from build123d import *

# Parameters (mm, degrees)
F1_DEPTH = 2
F2_DEPTH = 19
F3_R     = 2.75
F3_R_2   = 1.25
F4_DEPTH = 5
F5_W     = 9
F5_H     = 2
F5_W_2   = 17
F5_W_3   = 8
F5_W_4   = 2
F5_H_2   = 15.9
F5_H_3   = 15.1
F6_DEPTH = 12
F7_W     = 15.6
F7_H     = 4
F8_DEPTH = 2


with BuildPart() as f1:
    # F0 (on Top) → F1 (new body)
    with BuildSketch(Plane.XY):
        with BuildLine():
            ThreePointArc((0, 2.5), (0.732233047, 0.732233047), (2.5, 0))
            Line((2.5, 0), (88.5, 0))
            ThreePointArc((88.5, 0), (90.267766953, 0.732233047), (91, 2.5))
            Line((91, 2.5), (91, 59.5))
            ThreePointArc((91, 59.5), (90.267766953, 61.267766953), (88.5, 62))
            Line((88.5, 62), (2.5, 62))
            ThreePointArc((2.5, 62), (0.732233047, 61.267766953), (0, 59.5))
            Line((0, 59.5), (0, 2.5))
        make_face()
        with BuildLine():
            ThreePointArc((2, 59.5), (2.1464466094, 59.8535533906), (2.5, 60))
            Line((2.5, 60), (88.5, 60))
            ThreePointArc((88.5, 60), (88.8535533906, 59.8535533906), (89, 59.5))
            Line((89, 59.5), (89, 2.5))
            ThreePointArc((89, 2.5), (88.8535533906, 2.1464466094), (88.5, 2))
            Line((88.5, 2), (2.5, 2))
            ThreePointArc((2.5, 2), (2.1464466094, 2.1464466094), (2, 2.5))
            Line((2, 2.5), (2, 59.5))
        make_face(mode=Mode.SUBTRACT)
        with BuildLine():
            Line((88.5, 60), (2.5, 60))
            ThreePointArc((2.5, 60), (2.1464466094, 59.8535533906), (2, 59.5))
            Line((2, 59.5), (2, 2.5))
            ThreePointArc((2, 2.5), (2.1464466094, 2.1464466094), (2.5, 2))
            Line((2.5, 2), (88.5, 2))
            ThreePointArc((88.5, 2), (88.8535533906, 2.1464466094), (89, 2.5))
            Line((89, 2.5), (89, 59.5))
            ThreePointArc((89, 59.5), (88.8535533906, 59.8535533906), (88.5, 60))
        make_face()
    extrude(amount=F1_DEPTH)

    # F0 (on Top) → F2 (join)
    with BuildSketch(Plane.XY):
        with BuildLine():
            ThreePointArc((0, 2.5), (0.732233047, 0.732233047), (2.5, 0))
            Line((2.5, 0), (88.5, 0))
            ThreePointArc((88.5, 0), (90.267766953, 0.732233047), (91, 2.5))
            Line((91, 2.5), (91, 59.5))
            ThreePointArc((91, 59.5), (90.267766953, 61.267766953), (88.5, 62))
            Line((88.5, 62), (2.5, 62))
            ThreePointArc((2.5, 62), (0.732233047, 61.267766953), (0, 59.5))
            Line((0, 59.5), (0, 2.5))
        make_face()
        with BuildLine():
            ThreePointArc((2, 59.5), (2.1464466094, 59.8535533906), (2.5, 60))
            Line((2.5, 60), (88.5, 60))
            ThreePointArc((88.5, 60), (88.8535533906, 59.8535533906), (89, 59.5))
            Line((89, 59.5), (89, 2.5))
            ThreePointArc((89, 2.5), (88.8535533906, 2.1464466094), (88.5, 2))
            Line((88.5, 2), (2.5, 2))
            ThreePointArc((2.5, 2), (2.1464466094, 2.1464466094), (2, 2.5))
            Line((2, 2.5), (2, 59.5))
        make_face(mode=Mode.SUBTRACT)
    extrude(amount=F2_DEPTH)

    # F3 (on face) → F4 (join)
    with BuildSketch(Plane.XY.offset(2)):
        with Locations((6.5, 55.5)):
            Circle(F3_R)
        with Locations((6.5, 55.5)):
            Circle(F3_R_2, mode=Mode.SUBTRACT)
        with Locations((64.5, 55.5)):
            Circle(F3_R)
        with Locations((64.5, 55.5)):
            Circle(F3_R_2, mode=Mode.SUBTRACT)
        with Locations((6.5, 6.5)):
            Circle(F3_R)
        with Locations((6.5, 6.5)):
            Circle(F3_R_2, mode=Mode.SUBTRACT)
        with Locations((64.5, 6.5)):
            Circle(F3_R)
        with Locations((64.5, 6.5)):
            Circle(F3_R_2, mode=Mode.SUBTRACT)
    extrude(amount=F4_DEPTH)

    # F5 (on face) → F6 (cut)
    with BuildSketch(Plane.XY.offset(19)):
        with Locations((13.55, 1)):
            Rectangle(F5_W, F5_H)
        with Locations((35, 1)):
            Rectangle(F5_W_2, F5_H)
        with Locations((57.25, 1)):
            Rectangle(F5_W_3, F5_H)
        with Locations((90, 13.25)):
            Rectangle(F5_W_4, F5_H_2)
        with Locations((90, 30.95)):
            Rectangle(F5_W_4, F5_H_3)
        with Locations((90, 49.95)):
            Rectangle(F5_W_4, F5_H_3)
    extrude(amount=-F6_DEPTH, mode=Mode.SUBTRACT)

    # F7 (on face) → F8 (cut)
    with BuildSketch(Plane(origin=(0, 0, 0), x_dir=(0, -1, 0), z_dir=(-1, 0, 0))):
        with Locations((-31.7, 6)):
            Rectangle(F7_W, F7_H)
    extrude(amount=-F8_DEPTH, mode=Mode.SUBTRACT)


solid = f1.part
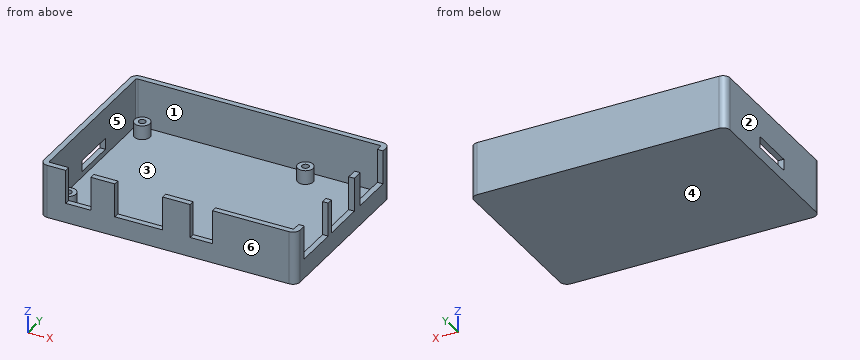
Read the model definition and answer for the solid it produces. Units are mm, in the model's axes. Face numbers are marked on the shaded views. A direction names the side the tool comes from. Give positions to 0.01 mm unless a question says otherwise; leave off trailing zeros. Write each loop counter-clockwise with the first axis right and the second up, starting at its lowest first coordinate (ties: lowest second). Pieces come first, ordered by that corner, then holes. Notation, with made-up numbers: (77.5, 77) -> (98.5, 77) arc R36 cw to (98.5, 111) -> close; hole circle Ø10 at (-7.75, 33). An arc over 180 degrees is marked (long way). Answer as a JSON object with one key per item and string values. Group by question number.
1) Find section A-A (y = 6.5). Write down the section's boundary in (x, z), and give its area (3 significant figures).
2) Each of these flat-tipped pins is pushed along its axis until it touches: P1, Ø2, axis at x = 35.5, y = 1, coming from the +Z side; P2, Ø1, axis at x = 90.5, z = 14.5, coming from the -Y side; P3, Ø0.6, axis at x = 89.5, z = 12, coming from the +Y side. Where does it stop, or does it pass through?
3) Find section D-D (y = 19.5). Write down the section's boundary in (x, z), and give its area (3 significant figures).
4) Consider L1, parallel to Y at x = 6.5, z = 4.8; L2, parallel to Y at x = 74, z = 2.5; L3, parallel to X at y = 58.5, z = 14.25. Determine where each line is inside the solid, lowest interval first. Write a range as from..to.
5) Find section B-B (x = 64.5). Write down the section's boundary in (y, z).
6) The mould has two halves that part along X. Classify the marked faces 1, 2, 3 and 4: +X half, -X half, draft (parallel to the pull), parting line (faces both ways), or undercut.
7) A tool of negligible diameter and unlimited length cuts with its end or side. For the marked faces 5 and 6, from which of +Z, -Z, +X, -X, +Y, -Y can it reach the whole face along a straight path? Write none if from no direction.
8) Find section C-C (z = 13). Count the separate pieces of the cut face and the enclosed holes in it, and give its area (3 significant figures).
Values follow:
{
 "1": {"outline": "(0, 0) -> (91, 0) -> (91, 7) -> (89, 7) -> (89, 2) -> (67.25, 2) -> (67.25, 7) -> (65.75, 7) -> (65.75, 2) -> (63.25, 2) -> (63.25, 7) -> (61.75, 7) -> (61.75, 2) -> (9.25, 2) -> (9.25, 7) -> (7.75, 7) -> (7.75, 2) -> (5.25, 2) -> (5.25, 7) -> (3.75, 7) -> (3.75, 2) -> (2, 2) -> (2, 19) -> (0, 19) -> close", "area": "256 mm2"},
 "2": {"P1": "stops at z = 7", "P2": "stops at y = 0.5", "P3": "stops at y = 61.9"},
 "3": {"outline": "(0, 0) -> (91, 0) -> (91, 7) -> (89, 7) -> (89, 2) -> (2, 2) -> (2, 19) -> (0, 19) -> close", "area": "226 mm2"},
 "4": {"L1": "y = 0..2, 3.75..5.25, 7.75..9.25, 52.75..54.25, 56.75..58.25, 60..62", "L2": "y = 0..2, 60..62", "L3": "x = 0..2, 89..91"},
 "5": {"outline": "(0, 0) -> (62, 0) -> (62, 19) -> (60, 19) -> (60, 2) -> (58.25, 2) -> (58.25, 7) -> (56.75, 7) -> (56.75, 2) -> (54.25, 2) -> (54.25, 7) -> (52.75, 7) -> (52.75, 2) -> (9.25, 2) -> (9.25, 7) -> (7.75, 7) -> (7.75, 2) -> (5.25, 2) -> (5.25, 7) -> (3.75, 7) -> (3.75, 2) -> (2, 2) -> (2, 19) -> (0, 19) -> close"},
 "6": {"face 1": "undercut", "face 2": "-X half", "face 3": "undercut", "face 4": "draft"},
 "7": {"face 5": "+Z", "face 6": "+Z, -Z, +X, -X, -Y"},
 "8": {"separate pieces": "6", "enclosed holes": "0", "area": "431 mm2"}
}
